Part model, mm, in its own coordinate system. A direction names the side the tool comes from. Round coordinates to 2 decimals unless told otherwise and drop trailing zeros. Write each loop counter-clockwise with the first axis right and the second up, starting at its lowest first coordinate (ties: lowest second). Pieces come first, ordered by that corner, then holes. Notation, with made-up numbers: M 73,80.25 L 101,80.25 A20 ccw 101,117.25 Z; hole C 70,12.25 d1. An arc over 180 degrees is marked long. Use a Markdown table: item, result. Add a question column.
1) Wall check: probe 1 along Y at (x, z) = (4.75, 1.25); probe 2 along X at (y, z) = (12.25, 7); probe 3 along Z at (x, y) = (1, 1.5). Give the ranges that are in metal, low to high.
2) Slice it at B-B on y = 7.25. Write the cut outline in (x, z), plus the area to 3 significant figures.
3) Slice it at A-A on x = 18.75. Write the cut outline in (y, z), plus the area to 4 significant figures.
4) Two-plate mould, pull along X, no slides. Class faces 1 (the face through (0, 11, 1)), 2 (the face through (13, 7, 1.9)), 3 (the face through (3, 7.3, 1)), 4 (the face through (24, 21, 3)): released by +X, released by -X, zero draft, split by the parting line, or undercut.
5) Which spindle directions (+Z, -Z, +X, -X, +Y, -Y) get a long thin tool onto all of the face, cutting with end or side? Do faces 5 (the face through (27, 16.5, 7)), 6 (the face through (7.434, 10.55, 10.086)), 7 (the face through (13.566, 18.45, 10.086)), 8 (the face through (15.454, 13.82, 10.086)). Say none if no direction does.
6) Slice it at C-C on z = 27. Write the cut outline in (x, y), plus the area to 3 significant figures.
7) Drop flat-ended pins along their axis: P1, Ø4, axis at x = 10.5, z = 8, coming from the +Y side; P2, Ø2, axis at x = 13, z = 7, coming from the +Y side; P3, Ø1, axis at y = 9, z = 8, coming from the -X side. Give the stop position or say it passes through.
8) Slice it at D-D on y = 19.5. Write the cut outline in (x, z), plus the area to 3 significant figures.
```python
from build123d import *

# Parameters (mm, degrees)
F0_W      = 26
F0_H      = 23
F1_DEPTH  = 1.9
F3_W      = 13
F3_H      = 11
F4_DEPTH  = 7
F5_R      = 6
F6_DEPTH  = 0.2
F8_DEPTH  = 2
F14_W     = 6.9831185974
F14_H     = 2.036742866
F15_DEPTH = 12
F16_SIZE  = 1
F17_W     = 2.5
F17_H     = 13
F18_DEPTH = 3
F20_R     = 1.75
F21_DEPTH = 2
F23_W     = 0.5
F23_H     = 0.5
F27_DEPTH = 0.5
F30_DEPTH = 0.5
F33_DEPTH = 0.5
F36_DEPTH = 0.5


with BuildPart() as f1:
    # F0 (on Top) → F1 (new body)
    with BuildSketch(Plane.XY):
        with Locations((13, 11.5)):
            Rectangle(F0_W, F0_H)
    extrude(amount=F1_DEPTH)

    # F3 (on face) → F4 (join)
    with BuildSketch(Plane.XY.offset(1.9)):
        with Locations((10.5, 14.5)):
            Rectangle(F3_W, F3_H)
    extrude(amount=F4_DEPTH)

    # F5 (on face) → F6 (join)
    with BuildSketch(Plane.XY.offset(8.9)):
        with Locations((10.5, 14.5)):
            Circle(F5_R)
    extrude(amount=F6_DEPTH)

    # F7 (on face) → F8 (join)
    with BuildSketch(Plane.XY.offset(9.1)):
        Polygon((5.1715213938, 12.277242911), (9.7607248024, 8.774023619), (15.0892034086, 10.996780708), (15.8284786062, 16.722757089), (11.2392751976, 20.225976381), (5.9107965914, 18.003219292), align=None)
    extrude(amount=F8_DEPTH)

    # F10 (on offset) → F11 (revolve)
    with BuildSketch(Plane(origin=(0, 14.5, 0), x_dir=(-1, 0, 0), z_dir=(0, 1, 0))):
        Polygon((-7.5, 11.1), (-7, 11.6), (-7.5, 12.1), (-7, 12.6), (-7.5, 13.1), (-7, 13.6), (-7.5, 14.1), (-7, 14.6), (-7.5, 15.1), (-10.5, 15.1), (-10.5, 11.1), align=None)
    revolve(axis=Axis((10.5, 14.5, 17.7832646295), (0, 0, -1)))

    # F12 (on offset) → F13 (revolve)
    with BuildSketch(Plane(origin=(0, 14.5, 0), x_dir=(-1, 0, 0), z_dir=(0, 1, 0))):
        Polygon((-7.5, 35.1), (-10.5, 35.1), (-10.5, 15.1), (-9, 15.1), (-9, 16.1), (-7.5, 16.1), align=None)
    revolve(axis=Axis((10.5, 14.5, 21.5967431704), (0, 0, -1)))

    # F14 (on face) → F15 (cut)
    with BuildSketch(Plane.XY.offset(35.1)):
        with Locations((10.4028915521, 11.8824467063)):
            Rectangle(F14_W, F14_H)
    extrude(amount=-F15_DEPTH, mode=Mode.SUBTRACT)

    # F16
    f16_edges = [f1.edges().sort_by_distance(p)[0] for p in [
        (11.332258, 17.382247, 35.1),
    ]]
    chamfer(f16_edges, length=F16_SIZE)

    # F17 (on face) → F18 (join)
    with BuildSketch(Plane.XY.offset(1.9)):
        with Locations((23.75, 14.5)):
            Rectangle(F17_W, F17_H)
    extrude(amount=F18_DEPTH)

    # F20 (on face) → F21 (cut)
    with BuildSketch(Plane.XY.offset(1.9)):
        with Locations((4.75, 7.25)):
            Circle(F20_R)
        with Locations((18.75, 7.25)):
            Circle(F20_R)
    extrude(amount=-F21_DEPTH, mode=Mode.SUBTRACT)

    # F24: sweep along a path in F22
    with BuildLine(Plane.XZ.offset(-9.25)) as f24_path:
        Line((23.75, 4.9), (23.75, 6.4))
        ThreePointArc((23.75, 6.4), (23.8964466094, 6.7535533906), (24.25, 6.9))
        Line((24.25, 6.9), (31.75, 6.9))
    # F23 (on face) → F24 (sweep)
    with BuildSketch(Plane.XY.offset(4.9)):
        with Locations((23.75, 9.25)):
            Rectangle(F23_W, F23_H)
    sweep(path=f24_path.line)

    # F26 (on offset) → F27 (join)
    with BuildSketch(Plane.XZ.offset(-11.5)):
        with BuildLine():
            Line((23.5, 6.4), (23.5, 4.9))
            Line((23.5, 4.9), (24, 4.9))
            Line((24, 4.9), (24, 6.4))
            ThreePointArc((24, 6.4), (24.0732233047, 6.5767766953), (24.25, 6.65))
            Line((24.25, 6.65), (31.75, 6.65))
            Line((31.75, 6.65), (31.75, 7.15))
            Line((31.75, 7.15), (24.25, 7.15))
            ThreePointArc((24.25, 7.15), (23.7196699141, 6.9303300859), (23.5, 6.4))
        make_face()
    extrude(amount=-F27_DEPTH)

    # F29 (on offset) → F30 (join)
    with BuildSketch(Plane.XZ.offset(-13.75)):
        with BuildLine():
            Line((23.5, 6.4), (23.5, 4.9))
            Line((23.5, 4.9), (24, 4.9))
            Line((24, 4.9), (24, 6.4))
            ThreePointArc((24, 6.4), (24.0732233047, 6.5767766953), (24.25, 6.65))
            Line((24.25, 6.65), (31.75, 6.65))
            Line((31.75, 6.65), (31.75, 7.15))
            Line((31.75, 7.15), (24.25, 7.15))
            ThreePointArc((24.25, 7.15), (23.7196699141, 6.9303300859), (23.5, 6.4))
        make_face()
    extrude(amount=-F30_DEPTH)

    # F32 (on offset) → F33 (join)
    with BuildSketch(Plane.XZ.offset(-16)):
        with BuildLine():
            Line((31.75, 7.15), (24.25, 7.15))
            ThreePointArc((24.25, 7.15), (23.7196699141, 6.9303300859), (23.5, 6.4))
            Line((23.5, 6.4), (23.5, 4.9))
            Line((23.5, 4.9), (24, 4.9))
            Line((24, 4.9), (24, 6.4))
            ThreePointArc((24, 6.4), (24.0732233047, 6.5767766953), (24.25, 6.65))
            Line((24.25, 6.65), (31.75, 6.65))
            Line((31.75, 6.65), (31.75, 7.15))
        make_face()
    extrude(amount=-F33_DEPTH)

    # F35 (on offset) → F36 (join)
    with BuildSketch(Plane.XZ.offset(-18.25)):
        with BuildLine():
            ThreePointArc((24, 6.4), (24.0732233047, 6.5767766953), (24.25, 6.65))
            Line((24.25, 6.65), (31.75, 6.65))
            Line((31.75, 6.65), (31.75, 7.15))
            Line((31.75, 7.15), (24.25, 7.15))
            ThreePointArc((24.25, 7.15), (23.7196699141, 6.9303300859), (23.5, 6.4))
            Line((23.5, 6.4), (23.5, 4.9))
            Line((23.5, 4.9), (24, 4.9))
            Line((24, 4.9), (24, 6.4))
        make_face()
    extrude(amount=-F36_DEPTH)


solid = f1.part
```
Entries:
| question | item | result |
|---|---|---|
| 1 | probe 1 | y = 0 to 5.5, 9 to 23 |
| 1 | probe 2 | x = 4 to 17 |
| 1 | probe 3 | z = 0 to 1.9 |
| 2 | outline | M 0,0 L 3,0 L 3,1.9 L 0,1.9 Z; M 6.5,0 L 17,0 L 17,1.9 L 6.5,1.9 Z; M 20.5,0 L 26,0 L 26,1.9 L 20.5,1.9 Z |
| 2 | area | 36.1 mm^2 |
| 3 | outline | M 0,0 L 5.5,0 L 5.5,1.9 L 0,1.9 Z; M 9,0 L 23,0 L 23,1.9 L 9,1.9 Z |
| 3 | area | 37.05 mm^2 |
| 4 | face 1 | released by -X |
| 4 | face 2 | undercut |
| 4 | face 3 | undercut |
| 4 | face 4 | zero draft |
| 5 | face 5 | +Z, +X |
| 5 | face 6 | +Z, -X, -Y |
| 5 | face 7 | +Z, +X, +Y |
| 5 | face 8 | +Z, +X, -Y |
| 6 | outline | M 7.96,12.9 L 13.04,12.9 A3 ccw long Z |
| 6 | area | 23.3 mm^2 |
| 7 | P1 | stops at y = 20.5 |
| 7 | P2 | stops at y = 20 |
| 7 | P3 | stops at x = 4 |
| 8 | outline | M 0,0 L 26,0 L 26,1.9 L 25,1.9 L 25,4.9 L 22.5,4.9 L 22.5,1.9 L 17,1.9 L 17,8.9 L 13.82,8.9 L 13.82,9.1 L 12.19,9.1 L 12.19,11.1 L 9.5,11.1 L 9.5,9.1 L 7.18,9.1 L 7.18,8.9 L 4,8.9 L 4,1.9 L 0,1.9 Z |
| 8 | area | 155 mm^2 |
